from build123d import *

# Parameters (mm, degrees)
SKETCH_R        = 2
PAD_DEPTH       = 42
SKETCH001_W     = 40
SKETCH001_H     = 7
POCKET_DEPTH    = 40
POCKET001_DEPTH = 5
SKETCH003_R     = 2
POCKET002_DEPTH = 5
FILLET_R        = 2


with BuildPart() as part:
    # Sketch → Pad (new body)
    with BuildSketch(Plane.XY):
        Polygon((0, 0), (38.845299, 0), (58.845299, -34.641016), (60.57735, -33.641016), (40, 2), (40, 9), (0, 9), align=None)
        with Locations((5, 5.5)):
            Circle(SKETCH_R, mode=Mode.SUBTRACT)
        with Locations((35, 5.5)):
            Circle(SKETCH_R, mode=Mode.SUBTRACT)
    extrude(amount=PAD_DEPTH)

    # Sketch001 (on Face11 of Pad) → Pocket (cut)
    with BuildSketch(Plane.XY.offset(42)):
        with Locations((20, 5.5)):
            Rectangle(SKETCH001_W, SKETCH001_H)
    extrude(amount=-POCKET_DEPTH, mode=Mode.SUBTRACT)

    # Sketch002 (on Face6 of Pocket) → Pocket001 (cut)
    with BuildSketch(Plane.XZ):
        Polygon((0, 2), (0, 42), (38.845299, 42), align=None)
    extrude(amount=-POCKET001_DEPTH, mode=Mode.SUBTRACT)

    # Sketch003 (on Face9 of Pocket001) → Pocket002 (cut)
    with BuildSketch(Plane(origin=(30.866025, 17.820508, 0), x_dir=(-0.5, 0.866025, 0), z_dir=(0.866025, 0.5, 0))):
        with Locations((-55.42265, 38)):
            Circle(SKETCH003_R)
        with Locations((-23.42265, 38)):
            Circle(SKETCH003_R)
        with Locations((-23.42265, 6)):
            Circle(SKETCH003_R)
        with Locations((-55.42265, 6)):
            Circle(SKETCH003_R)
        Polygon((-21.42265, 29.455844), (-31.966806, 40), (-46.878494, 40), (-57.42265, 29.455844), (-57.42265, 14.544156), (-46.878494, 4), (-31.966806, 4), (-21.42265, 14.544156), align=None)
    extrude(amount=-POCKET002_DEPTH, mode=Mode.SUBTRACT)

    # Fillet
    fillet_edges = [part.edges().sort_by_distance(p)[0] for p in [
        (59.711325, -34.141016, 42),
        (59.711325, -34.141016, 0),
        (40, 9, 1),
        (0, 9, 1),
    ]]
    fillet(fillet_edges, radius=FILLET_R)


solid = part.part
Geometry check sheet. Reference: the model listing, model coordinates, mm. A direction names the side the tool comes from. Round coordinates to 2 decimals unless told otherwise and drop trailing zeros. Order: outer loops, then holes, each group sorted by start corner. A loop starts at its lowest first (then second) coordinate and runs counter-clockwise, first axis right, second up. Notation, with made-up numbers: M 47.25,48.5 L 89.25,48.5 A31 cw 89.25,77.5 Z; hole C -32.5,34 d8. An arc over 180 degrees is marked long. Answer in a Markdown table with one row per item.
(1) Tool access check on faces 5 (the face through (56.124, -27.9, 9.346)), 6 (the face through (43.323, -5.727, 34.654)), 7 (the face through (41.94, -3.333, 36.048)), 8 (the face through (40, 4, 1)), 9 (the face through (20, 6, 2)). Record the directions out of +Z, -Z, +X, -X, +Y, -Y that give a thin tool (end or side, any length) a straight path to the whole face; none if there is none.
Responses:
| item | result |
|---|---|
| face 5 | -X, +Y |
| face 6 | +X, -Y |
| face 7 | none |
| face 8 | +Z, -Z, +X, +Y |
| face 9 | +Z, +X, -X, +Y |
(2) Sectioned sample at D-D, the plane y = -27. Record the cut outline in (x, z), and give its area (3 significant figures).
Responses:
| item | result |
|---|---|
| outline | M 54.43,0 L 56.74,0 L 56.74,8.88 L 54.43,7.72 Z; M 54.43,36.28 L 56.74,35.12 L 56.74,42 L 54.43,42 Z |
| area | 33.7 mm² |
(3) Scan lines: probe 1 along X at (y, z) = (5.5, 0.5); probe 2 along Y at (x, z) = (35, 1); probe 3 along X at (y, z) = (5, 1). Record each from-to range of solid material in increasing order. Write a range as from..to.
Responses:
| item | result |
|---|---|
| probe 1 | x = 0..3, 7..33, 37..40 |
| probe 2 | y = 0..3.5, 7.5..9 |
| probe 3 | x = 0..3.06, 6.94..33.06, 36.94..40 |
(4) Go/stop test with flat-tipped pins: P1, Ø1, axis at x = 41.5, z = 15.5, coming from the +Y side; P2, Ø5, axis at x = 35, y = 5.5, coming from the -Z side; P3, Ø19.5, axis at x = 18.5, z = 28, coming from the -Y side; P4, Ø20, axis at x = 23.5, z = 30.5, coming from the +Y side. Record where each tip stops, or that it passes through.
Responses:
| item | result |
|---|---|
| P1 | stops at y = 0.27 |
| P2 | stops at z = 0 |
| P3 | stops at y = 0 |
| P4 | stops at y = 2 |
(5) Draft check along Y on faces 1 (the face through (42.7, -4.7, 6.1)), 2 (the face through (59.423, -33.613, 0.57)), 3 (the face through (50.433, -16.07, 2.039)), 4 (the face through (25, 1, 0)). Enter one of: released by +Y, released by -Y, zero draft, split by the parting line, or undercut.
Responses:
| item | result |
|---|---|
| face 1 | undercut |
| face 2 | released by -Y |
| face 3 | released by +Y |
| face 4 | zero draft |
(6) Sectioned sample at C-C, the plane x = 35. Record the cut outline in (y, z).
Responses:
| item | result |
|---|---|
| outline | M 0,0 L 3.5,0 L 3.5,2 L 2,2 L 2,38.04 L 0,38.04 Z; M 7.5,0 L 9,0 L 9,2 L 7.5,2 Z |
(7) Sectioned sample at A-A, the plane y = 5.5. Record the cut outline in (x, z), and give its area (3 significant figures).
Responses:
| item | result |
|---|---|
| outline | M 0,0 L 3,0 L 3,2 L 0,2 Z; M 7,0 L 33,0 L 33,2 L 7,2 Z; M 37,0 L 40,0 L 40,2 L 37,2 Z |
| area | 64.0 mm² |
(8) Sectioned sample at B-B, the plane z = 33.5. Record the cut outline in (x, y), and give its area (3 significant figures).
Responses:
| item | result |
|---|---|
| outline | M 30.59,0 L 38.85,0 L 41.87,-5.23 L 43.6,-4.23 L 40,2 L 30.59,2 Z; M 55.82,-29.41 L 58.85,-34.64 L 60.58,-33.64 L 57.56,-28.41 Z |
| area | 43.0 mm² |
